Part model, mm, in its own coordinate system. A direction names the side the tool comes from. Round coordinates to 2 decimals unless told otherwise and drop trailing zeros. Write each loop counter-clockwise with the first axis right and the second up, starting at its lowest first coordinate (ties: lowest second). Pieces come first, ordered by that corner, then holes.
Autodesk Inventor part; units mm, degrees
ref_plane "YZ Plane" through (0, 0, 0) normal (1, 0, 0) x (0, 1, 0)
ref_plane "XZ Plane" through (0, 0, 0) normal (0, 1, 0) x (-1, 0, 0)
ref_plane "XY Plane" through (0, 0, 0) normal (0, 0, 1) x (1, 0, 0)
sketch "Sketch1" plane through (0, 0, 0) normal (0, 1, 0) x (-1, 0, 0)
  circle A0 centre (-8.5046, 0.0113) radius 2
  circle A1 centre (0.0454, 0.0113) radius 12.5
  circle A2 centre (-8.5046, 0.0113) radius 1.5
  circle A3 centre (8.5954, 0.0113) radius 2
  circle A4 centre (8.5954, 0.0113) radius 1.5
  circle A5 centre (0.0454, 0.0113) radius 3.5
  line L0 (-12.4546, 0.0113) -> (12.5454, 0.0113)
  line L1 (12.5454, 17.5113) -> (-12.4546, 17.5113)
  circle A6 centre (0.0454, 0.0113) radius 14.5
  line L2 (-12.4546, 17.5113) -> (-14.3509, 1.7426)
  line L3 (12.5454, 17.5113) -> (14.4417, 1.7426)
  circle A7 centre (0.0454, 0.0113) radius 12.8
  point P0 (0, 0)
  dimension "d0" = 17.5
  dimension "d2" = 2
  dimension "d5" = 0.3
extrude "Extrusion1" add sketch "Sketch1" along normal blind 2.6 contours L0 A5 A3 A1 A0 | A0 L0 A1 A3 A5 | L3 A6 L2 L1 | A6 | A7
extrude "Extrusion2" add sketch "Sketch1" against normal blind 25 contours L3 A6 L2 L1 | A6
sketch "Sketch2" plane through (-12.5454, 2.6, 17.5113) normal (0, 0, 1) x (1, 0, 0)
  line L0 (25, -27.6) -> (0, -27.6) construction
  line L1 (25, -27.6) -> (0, 0) construction
  line L2 (0, -27.6) -> (25, 0) construction
  line L3 (27, 0) -> (-2, 0) construction
  line L4 (19.4, -13.8) -> (5.6, -13.8) construction
  point P0 (12.5454, -2.6)
  point P1 (26.8963, 0)
  point P2 (-1.8963, 0)
  point P3 (12.5, -13.8)
  dimension "d8" = 13.8
hole "Hole1" at (6.8546, -11.2, 17.5113) at (-6.9454, -11.2, 17.5113) direction (0, 0, -1) diameter 3 depth 12 tip angle 118 countersink diameter 4 countersink angle 90
fillet "Fillet1" radius 2 3 edges at (-0.0454, 2.6, -14.4887) (-13.4935, 2.6, 9.627) (13.4027, 2.6, 9.627)
properties part number "motor_holder"
Q1. Cut at A-A on y = -11.2. Write the cut outline in (x, z).
Values follow:
outline: (-14.44, 1.74) arc R14.5 ccw (long way) to (14.35, 1.74) - (12.45, 17.51) - (8.85, 17.51) - (8.35, 17.01) - (8.35, 9.67) arc R12.8 cw (long way) to (-8.45, 9.67) - (-8.45, 17.01) - (-8.95, 17.51) - (-12.55, 17.51) - close; (-5.45, 11.62) arc R12.8 cw to (5.35, 11.62) - (5.35, 17.01) - (4.85, 17.51) - (-4.95, 17.51) - (-5.45, 17.01) - close
Q2. Cut at B-B on x = -7.5. State how many separate pieces and enclosed holes the cut face has, plus the area to 3 significant figures.
Values follow:
separate pieces: 3
enclosed holes: 0
area: 276 mm2
Q3. Which spindle directions (+Z, -Z, +X, -X, +Y, -Y) get a long thin tool onto all of the face, cutting with end or side? Do faces 1 (the cylindrical face through (8.319, -10.875, 14.105)), 2 (the flat face through (-3, 0, -3)), 3 (the cylindrical face through (12.805, 2.03, 9.562)). Say none if no direction does.
Values follow:
face 1: +Z
face 2: -Y
face 3: +Z, +X, +Y
Q4. Drop flat-ended pins along their axis: pin 1 (6.5 mm diameter, centred on x = -0.05, z = 0.01, fed in from -Y); pin 2 (8 mm diameter, centred on x = -7, z = 1, fed in from -Y); pin 3 (2.5 mm diameter, centred on x = 6.85, y = -11.2, fed in from +Z); pin 4 (1 mm diameter, centred on y = -11, z = 6, fed in from +X). Give the stop position or say it passes through.
Values follow:
pin 1: passes through
pin 2: stops at y = 0
pin 3: stops at z = -9.86
pin 4: stops at x = 13.9
Q5. Wall check: L1, parallel to Z at x = -0.5, y = -8.5; L2, parallel to Y at x = -2.5, z = 7.5; L3, parallel to Z at x = -9.75, y = -13 (3 decimals). Give the ranges that are in metal, low to high.
Values follow:
L1: z = -14.48 to -12.78, 12.8 to 17.51
L2: y = 0 to 2.6
L3: z = -10.762 to -8.335, 8.358 to 17.511
Q6. Mould opens along Y. For faces 4 (the flat face through (0, 2.6, 6)), 5 (the cylindrical face through (-8.43, -11, 14.1)), 6 (the cylindrical face through (2.732, 1.282, 2.141)) say: +Y half, -Y half, draft (parallel to the pull), parting line (faces both ways), or undercut.
Values follow:
face 4: +Y half
face 5: undercut
face 6: draft
